```python
from build123d import *

# Parameters (mm, degrees)
BOSS_EXTRUDE1_DEPTH     = 25.4
FILLET1_R               = 3.81
FILLET2_R               = 3.81
CUT_EXTRUDE1_DEPTH      = 77.2
CUT_EXTRUDE1_DEPTH_BACK = 77.2
SKETCH2_R               = 3.556


with BuildPart() as part:
    # Sketch1 → Boss-Extrude1 (new, symmetric)
    with BuildSketch(Plane.XY):
        with BuildLine():
            Line((-19.05, 50.8), (-25.4, 50.8))
            Line((-25.4, 50.8), (-25.4, 0))
            ThreePointArc((-25.4, 0), (19.05, -16.800520825), (-3.175, 25.200781238))
            Line((-3.175, 25.200781238), (-3.175, 50.8))
            Line((-3.175, 50.8), (-9.525, 50.8))
            Line((-9.525, 50.8), (-9.525, 16.497783942))
            ThreePointArc((-9.525, 16.497783942), (16.497783942, -9.525), (-19.05, 0))
            Line((-19.05, 0), (-19.05, 50.8))
        make_face()
    extrude(amount=BOSS_EXTRUDE1_DEPTH, both=True)

    # Fillet1
    fillet1_edges = [part.edges().sort_by_distance(p)[0] for p in [
        (-9.525, 16.497783942, 0),
    ]]
    fillet(fillet1_edges, radius=FILLET1_R)

    # Fillet2
    fillet2_edges = [part.edges().sort_by_distance(p)[0] for p in [
        (-3.175, 25.200781238, 0),
    ]]
    fillet(fillet2_edges, radius=FILLET2_R)

    # Sketch2 → Cut-Extrude1 (cut, two sides: drawn at the far end of the back side and taken through both)
    with BuildSketch(Plane.ZY.offset(25.4).offset(-CUT_EXTRUDE1_DEPTH_BACK)):
        with Locations(Location((0, 41.148, 0), (0, 0, 270))):
            Circle(SKETCH2_R)
    extrude(amount=CUT_EXTRUDE1_DEPTH + CUT_EXTRUDE1_DEPTH_BACK, mode=Mode.SUBTRACT)


solid = part.part
```
Geometry: final body of the model. Coordinates: model frame, mm. A direction names the side the tool comes from. Coordinates: 2 decimals unless noted, no trailing zeros. Order: outer loops, then holes, each group sorted by start corner. A loop starts at its lowest first (then second) coordinate and runs counter-clockwise, first axis right, second up. Notation, with made-up numbers: M 69,87.5 L 91,87.5 A32 ccw 91,118.5 Z; hole C -19.75,75.5 d11. An arc over 180 degrees is marked long. Answer in a Markdown table with one row per item. Add a question column.
Q1. Section query B-B on z = -1. Count the separate pieces of the cut face and the enclosed holes in it, and give its area (3 significant figures).
Q2. Line query: L1, parallel to X at y = 41, z = -13 (3 decimals); L2, parallel to Y at x = -22, z = 0. Output: solid intervals per line, ascending.
Q3. Contact query for flat-ended pins moving along their axis: P1, Ø11, axis at y = 44.5, z = 11, coming from the +X side (3 decimals); P2, Ø11.5, axis at y = 41.148, z = 0, coming from the -X side; P3, Ø5, axis at y = 4.5, z = 19.5, coming from the +X side; P4, Ø6, axis at x = 18, z = 11.5, coming from the +Y side. Output: stop coordinate, or through.
Q4. Mould query, pull axis Y, two halves, no side actions, for faces 4 (the cylindrical face through (-8.01, 19.092, -0.356)), 5 (the flat face through (-22, 50.8, 0)), 6 (the flat face through (-25.4, 26, 0)). Classes: released by +Y, released by -Y, zero draft, split by the parting line, or undercut.
Q5. Section query C-C on x = 8.5. Return the cut outline in (y, z), and give its area (3 significant figures).
Q6. Reachability of faces 1 (the flat face through (-3.175, 37, 0)), 2 (the cylindrical face through (-6.306, 37.756, 1.068)), 3 (the flat face through (-19.05, 25, 0)) from +Z, -Z, +X, -X, +Y, -Y: full face, straight path, thin tool, end or side. Return the list, or none.
Q7. Section query A-A on y = 34. Return the cut outline in (x, z) (3 decimals), and give its area (3 significant figures).
Completed:
| question | item | result |
|---|---|---|
| 1 | separate pieces | 3 |
| 1 | enclosed holes | 0 |
| 1 | area | 1,130 mm2 |
| 2 | L1 | x = -25.4 to -19.05, -9.525 to -3.175 |
| 2 | L2 | y = -12.69 to 37.59, 44.7 to 50.8 |
| 3 | P1 | stops at x = -3.175 |
| 3 | P2 | stops at x = -25.4 |
| 3 | P3 | stops at x = 25.32 |
| 3 | P4 | stops at y = 20.5 |
| 4 | face 4 | undercut |
| 4 | face 5 | released by +Y |
| 4 | face 6 | zero draft |
| 5 | outline | M -23.94,-25.4 L -17.05,-25.4 L -17.05,25.4 L -23.94,25.4 Z; M 17.05,-25.4 L 23.94,-25.4 L 23.94,25.4 L 17.05,25.4 Z |
| 5 | area | 700 mm2 |
| 6 | face 1 | +Z, -Z, +X, +Y |
| 6 | face 2 | +X, -X |
| 6 | face 3 | +Z, -Z, +Y |
| 7 | outline | M -25.4,-25.4 L -19.05,-25.4 L -19.05,25.4 L -25.4,25.4 Z; M -9.525,-25.4 L -3.175,-25.4 L -3.175,25.4 L -9.525,25.4 Z |
| 7 | area | 645 mm2 |
